Source: three-view drawing plus pictorial views. Frame: mm from the lowest corner of the part. A direction names the side the tool comes from. Coordinates: 2 decimals unless noted, no trailing zeros. Order: outer loops, then holes, each group sorted by start corner. A loop starts at its lowest first (then second) coordinate and runs counter-clockwise, first axis right, second up. Notation, with made-up numbers: M 80.5,74.25 L 129.5,74.25 A14 cw 129.5,88.25 Z; hole C -9.75,45.25 d2. An arc over 180 degrees is marked long. One line per question, with ' | ' between items.
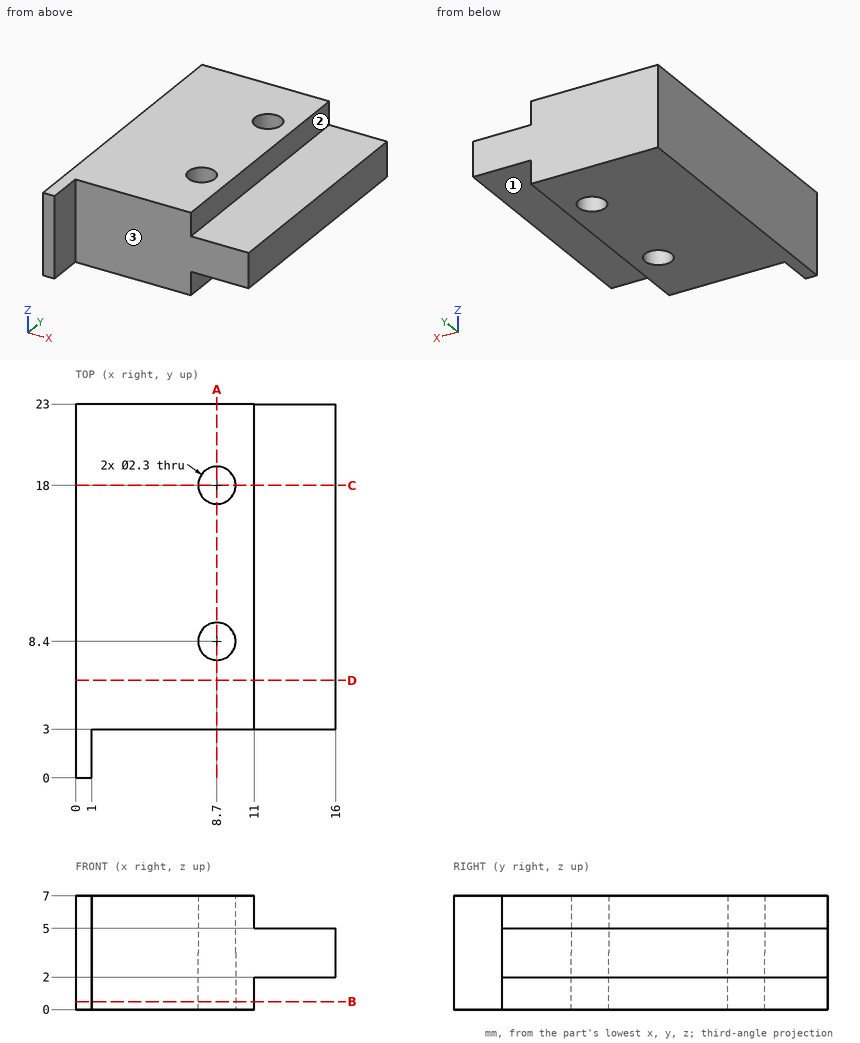
1. Material intervals for line 1 (Y direction, x = 8.7, z = 2.1); line 2 (Y direction, x = 8, z = 3.5); line 3 (Y direction, x = 5.5, z = 3.75), sorted ascending. Write a range as [from, to].
Response values:
line 1: y = [3, 7.25], [9.55, 16.85], [19.15, 23] | line 2: y = [3, 7.49], [9.31, 17.09], [18.91, 23] | line 3: y = [3, 23]
2. Pin query (flat end, axial travel): P1, Ø2.5, axis at x = 14, y = 8.5, coming from the -Z side; P2, Ø1.6, axis at y = 12.5, z = 6, coming from the +X side; P3, Ø4, axis at x = 13.5, y = 3.5, coming from the +Z side. Return the tip coordinate at first contact, or that it passes through.
Response values:
P1: stops at z = 2 | P2: stops at x = 11 | P3: stops at z = 5
3. Section B-B, the plane z = 0.5. Output: boundary loops of the cut face in (x, y).
Response values:
outline: M 0,0 L 1,0 L 1,3 L 11,3 L 11,23 L 0,23 Z; hole C 8.7,8.4 d2.3; hole C 8.7,18 d2.3
4. Section A-A, the plane x = 8.7. Output: boundary loops of the cut face in (y, z).
Response values:
outline: M 3,0 L 7.25,0 L 7.25,7 L 3,7 Z; M 9.55,0 L 16.85,0 L 16.85,7 L 9.55,7 Z; M 19.15,0 L 23,0 L 23,7 L 19.15,7 Z
5. Section C-C, the plane y = 18. Output: boundary loops of the cut face in (x, z).
Response values:
outline: M 0,0 L 7.55,0 L 7.55,7 L 0,7 Z; M 9.85,0 L 11,0 L 11,2 L 16,2 L 16,5 L 11,5 L 11,7 L 9.85,7 Z
6. Section D-D, the plane y = 6. Output: boundary loops of the cut face in (x, z), and give its area (3 significant figures).
Response values:
outline: M 0,0 L 11,0 L 11,2 L 16,2 L 16,5 L 11,5 L 11,7 L 0,7 Z | area: 92.0 mm^2
7. Access query for the marked faces 1, 2 and 3. Directions: +Z, -Z, +X, -X, +Y, -Y. A direction counts if a zero-diameter tool reaches every point of the face in a straight line with its end or side. Return the directions, or none.
Response values:
face 1: -Z, +X, +Y, -Y | face 2: +Z, +X, +Y, -Y | face 3: +Z, -Z, +X, -Y
